Geometry: final body of the model. Coordinates: model frame, mm. Face numbers are marked on the shaded views. A direction names the side the tool comes from. Give positions to 0.01 mm unless a question says otherwise; leave off trailing zeros. Loops run counter-clockwise (first coordinate to the right, second up) from the corner with the lowest first, then second, coordinate; pieces in that order, holes last.
1. Section C-C, the plane x = -2. Output: boundary loops of the cut face in (y, z).
2. Access query for the marked faces 4, 5, 6 and 7. Directions: +Z, -Z, +X, -X, +Y, -Y. A direction counts if a zero-diameter tool reaches every point of the face in a straight line with its end or side. Return the directions, or none.
3. Section A-A, the plane z = 12. Output: boundary loops of the cut face in (x, y), then the cut area to 3 significant figures.
4. Material intervals for line 1 along X through (y, z) = (-6.5, 8); line 2 along Y through (x, z) = (-30, 9.5); line 3 along X through (y, z) = (-27, 7), sorted ascending.
5. Section D-D, the plane z = 23.5. Output: boundary loops of the cut face in (x, y), then the cut area to 3 significant figures.
6. First-contact query: P1, Ø2.5, axis at x = -30, y = -27.5, coming from the -Z side; P2, Ø4, axis at y = 34, z = 21.5, coming from the -X side; P3, Ø12, axis at x = -8, z = 25.5, coming from the +Y side; P4, Ø6, axis at x = 0, y = 32, coming from the -Z side. Flat tips, straight axial feed; report the tip coordinate or a pass-through.
7. Section B-B, the plane y = -27.5. Output: boundary loops of the cut face in (x, z), then the cut area to 3 significant figures.
8. Draft query along X for the marked faces 1, 2 and 3. Return one class per face: +X half, -X half, draft (parallel to the pull), parting line (faces both ways), or undercut.
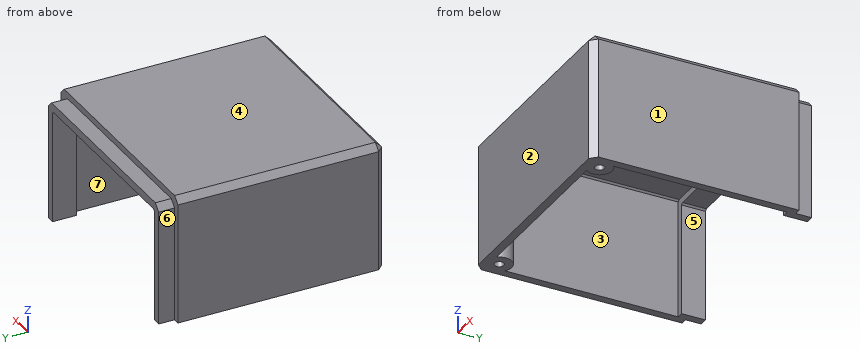
from build123d import *

# Parameters (mm, degrees)
F0_R        = 1.45
F0_W        = 66
F0_H        = 5
F1_DEPTH    = 40
F2_DEPTH    = 38
F3_SIZE     = 2
F4_T        = 2.5
F4_T3_DEPTH = 41
F4_T5_DEPTH = 7.8284271247
F4_T7_DEPTH = 67
F4_T9_DEPTH = 7.8284271247
F5_START    = 20
F5_DEPTH    = 20


# Not quite as in the source:
# - a shell that OpenCascade refuses in one call is made with other operations: the cavity is built on its own and cut out


with BuildPart() as f1:
    # F0 (on Top) → F1 (new body)
    with BuildSketch(Plane.XY):
        Polygon((-33, 32.5), (-35, 32.5), (-35, -32.5), (35, -32.5), (35, 32.5), (33, 32.5), (33, 27.5), (-33, 27.5), align=None)
        with Locations((-30, -27.5)):
            Circle(F0_R, mode=Mode.SUBTRACT)
        with Locations((30, -27.5)):
            Circle(F0_R, mode=Mode.SUBTRACT)
        with Locations((0, 30)):
            Rectangle(F0_W, F0_H)
    extrude(amount=F1_DEPTH)

    # F0 (on Top) → F2 (join)
    with BuildSketch(Plane.XY):
        Polygon((-33, 32.5), (-35, 32.5), (-35, -32.5), (35, -32.5), (35, 32.5), (33, 32.5), (33, 27.5), (-33, 27.5), align=None)
        with Locations((-30, -27.5)):
            Circle(F0_R, mode=Mode.SUBTRACT)
        with Locations((30, -27.5)):
            Circle(F0_R, mode=Mode.SUBTRACT)
        with Locations((0, 35)):
            Rectangle(F0_W, F0_H)
        with Locations((0, 30)):
            Rectangle(F0_W, F0_H)
    extrude(amount=F2_DEPTH)

    # F3
    f3_edges = [f1.edges().sort_by_distance(p)[0] for p in [
        (0, -32.5, 40),
        (35, 0, 40),
        (-35, 0, 40),
        (33, 35, 38),
        (-33, 35, 38),
        (-35, -32.5, 20),
        (35, -32.5, 20),
    ]]
    chamfer(f3_edges, length=F3_SIZE)

    # F4: shell of thickness 2.5, made by hand


with BuildPart() as f4_core1:
    # F4_t2: copy of F1
    add(f1.part)

    # the walls: a layer under each face that stays
    f4_faces = [f4_core1.faces().sort_by_distance(p)[0] for p in [
        (-35, 1, 19),
        (-34, -31.5, 19),
        (32.6666666667, 32.5, 38.6666666667),
        (-34, 1, 39),
        (0, -32.5, 19),
        (-33, 35, 18),
        (34, -31.5, 19),
        (35, 1, 19),
        (33, 35, 18),
        (-31.45, -27.5, 20),
        (28.55, -27.5, 20),
        (-34, -31, 38.5),
        (-32, 35, 37),
        (0, 35, 38),
        (32, 35, 37),
        (0, 1, 40),
        (34, 1, 39),
        (0, -31.5, 39),
        (34, -31, 38.5),
    ]]
    thicken(f4_faces, amount=-F4_T, mode=Mode.SUBTRACT)

    # F4_s4 → F4_t3 (cut)
    with BuildSketch(Plane.XY.offset(-2.5)):
        Polygon((-33.025, 32.525), (-33, 30), (-30.5, 30), (-30.5, 32.5), align=None)
        Polygon((33.025, 32.525), (33, 30), (30.5, 30), (30.5, 32.5), align=None)
    extrude(amount=F4_T3_DEPTH, mode=Mode.SUBTRACT)

    # F4_s6 → F4_t5 (cut)
    with BuildSketch(Plane(origin=(5.267766953, 0, 5.267766953), x_dir=(0, 1, 0), z_dir=(-0.7071067812, 0, -0.7071067812))):
        Polygon((32.525, -48.8153679019), (30, -48.7903679019), (30, -46.2903679019), (32.5, -46.2903679019), align=None)
    extrude(amount=F4_T5_DEPTH, mode=Mode.SUBTRACT)

    # F4_s8 → F4_t7 (cut)
    with BuildSketch(Plane.YZ.offset(-33.5)):
        Polygon((32.525, 38.025), (30, 38), (30, 35.5), (32.5, 35.5), align=None)
    extrude(amount=F4_T7_DEPTH, mode=Mode.SUBTRACT)

    # F4_s10 → F4_t9 (cut)
    with BuildSketch(Plane(origin=(0.267766953, 0, -0.267766953), x_dir=(0, 1, 0), z_dir=(-0.7071067812, 0, 0.7071067812))):
        Polygon((32.525, -48.8153679019), (30, -48.7903679019), (30, -46.2903679019), (32.5, -46.2903679019), align=None)
    extrude(amount=F4_T9_DEPTH, mode=Mode.SUBTRACT)


with BuildPart() as f1_1:
    add(f1.part)

    # what is left inside the walls is the cavity
    f4_cavity = [f4_core1.part.solids().sort_by_distance(p)[0] for p in [
        (0, -7.5, 0.025),
    ]]
    add(f4_cavity, mode=Mode.SUBTRACT)

    # F0 (on Top) → F5 (join)
    with BuildSketch(Plane.XY.offset(F5_START)):
        with Locations((-30, -27.5)):
            Circle(F0_R)
        with Locations((30, -27.5)):
            Circle(F0_R)
    extrude(amount=F5_DEPTH)


solid = f1_1.part
Answers below:
1. outline: (-32.5, 0) - (-30, 0) - (-30, 36.96) - (-29.46, 37.5) - (30, 37.5) - (30, 35.5) - (37.5, 35.5) - (37.5, 38) - (32.5, 38) - (32.5, 40) - (-30.5, 40) - (-32.5, 38) - close
2. face 4: +Z, +X, -X, +Y, -Y
2. face 5: -Z, +Y
2. face 6: +Z, -Z, -X, +Y
2. face 7: -Z
3. outline: (-35, -30.5) - (-33, -32.5) - (33, -32.5) - (35, -30.5) - (35, 32.5) - (33, 32.5) - (33, 37.5) - (30.5, 37.5) - (30.5, 30) - (32.5, 30) - (32.5, -24.44) arc R3.95 ccw to (26.94, -30) - (-26.94, -30) arc R3.95 ccw to (-32.5, -24.44) - (-32.5, 30) - (-30.5, 30) - (-30.5, 37.5) - (-33, 37.5) - (-33, 32.5) - (-35, 32.5) - close; hole circle Ø2.9 at (-30, -27.5); hole circle Ø2.9 at (30, -27.5)
3. area: 579 mm2
4. line 1: x = -35 to -32.5, 32.5 to 35
4. line 2: y = -32.5 to -28.95, -26.05 to -23.55
4. line 3: x = -35 to -31.36, -28.64 to -26.08, 26.08 to 28.64, 31.36 to 35
5. outline: (-35, -30.5) - (-33, -32.5) - (33, -32.5) - (35, -30.5) - (35, 32.5) - (33, 32.5) - (33, 37.5) - (30.5, 37.5) - (30.5, 30) - (32.5, 30) - (32.5, -24.44) arc R3.95 ccw to (26.94, -30) - (-26.94, -30) arc R3.95 ccw to (-32.5, -24.44) - (-32.5, 30) - (-30.5, 30) - (-30.5, 37.5) - (-33, 37.5) - (-33, 32.5) - (-35, 32.5) - close
5. area: 592 mm2
6. P1: stops at z = 20
6. P2: stops at x = -35
6. P3: stops at y = -30
6. P4: stops at z = 35.5
7. outline: (-35, 0) - (-31.45, 0) - (-31.45, 20) - (-28.55, 20) - (-28.55, 0) - (-26.05, 0) - (-26.05, 37.5) - (26.05, 37.5) - (26.05, 0) - (28.55, 0) - (28.55, 20) - (31.45, 20) - (31.45, 0) - (35, 0) - (35, 38) - (33, 40) - (-33, 40) - (-35, 38) - close
7. area: 726 mm2
8. face 1: +X half
8. face 2: draft
8. face 3: undercut
